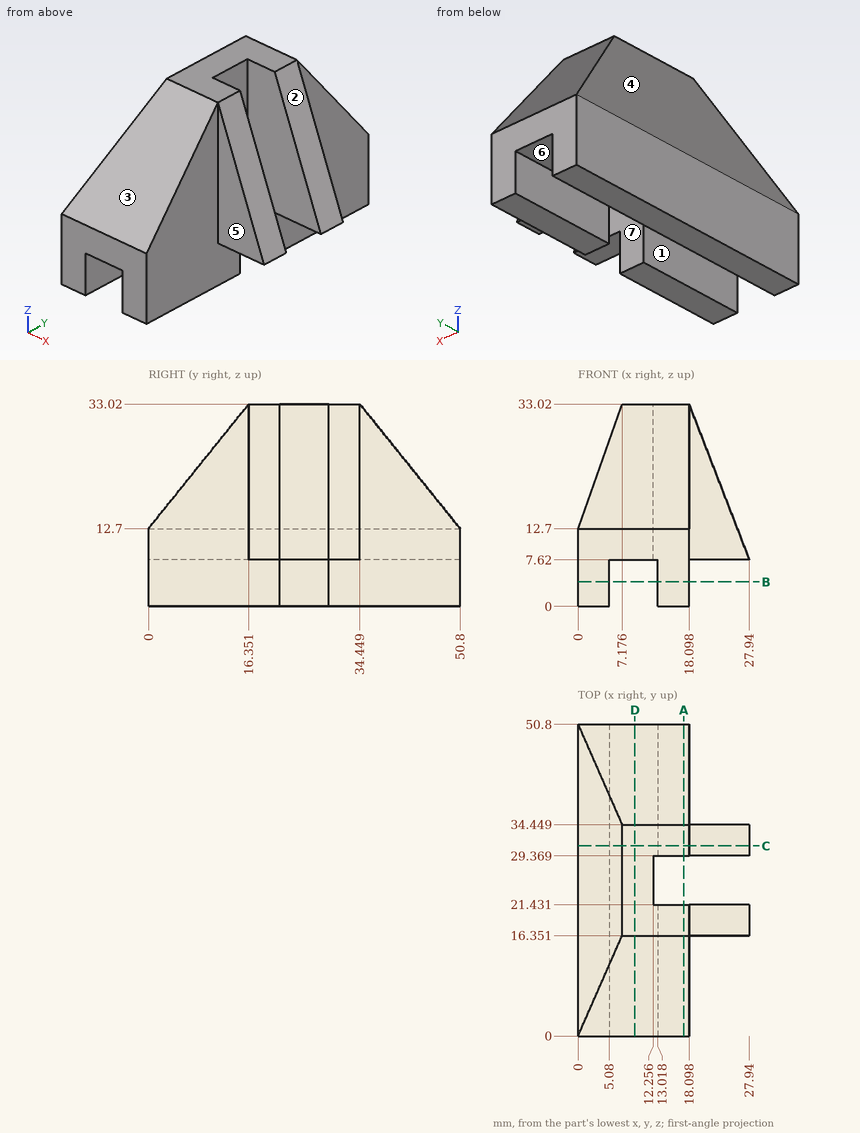
Geometry: see drawing. Coordinates: mm, zero at the bounding-box minimum. A direction names the side the tool comes from. Give positions to 0.01 mm unless a question says otherwise; leave off trailing zeros. Order: outer loops, then holes, each group sorted by start corner. A loop starts at its lowest first (then second) coordinate and runs counter-clockwise, first axis right, second up.
1. Cut plane B-B (z = 4). Return loops of the section in (x, y), and give its area (3 significant figures).
Computed:
outline: (0, 0) - (5.08, 0) - (5.08, 50.8) - (0, 50.8) - close; (13.02, 0) - (18.1, 0) - (18.1, 21.43) - (13.02, 21.43) - close; (13.02, 29.37) - (18.1, 29.37) - (18.1, 50.8) - (13.02, 50.8) - close
area: 476 mm2
2. Cut plane A-A (x = 17.25). Return loops of the section in (y, z).
Computed:
outline: (0, 0) - (21.43, 0) - (21.43, 33.02) - (16.35, 33.02) - (0, 12.7) - close; (29.37, 0) - (50.8, 0) - (50.8, 12.7) - (34.45, 33.02) - (29.37, 33.02) - close
3. Cut plane D-D (x = 9.25). Return loops of the section in (y, z).
Computed:
outline: (0, 7.62) - (50.8, 7.62) - (50.8, 12.7) - (34.45, 33.02) - (16.35, 33.02) - (0, 12.7) - close
4. Cut plane C-C (y = 31). Return loops of the section in (x, z) (1 decimal).
Computed:
outline: (0, 0) - (5.1, 0) - (5.1, 7.6) - (13, 7.6) - (13, 0) - (18.1, 0) - (18.1, 7.6) - (27.9, 7.6) - (18.1, 33) - (7.2, 33) - (0, 12.7) - close
5. Draft query along X for the marked faces 1, 2, 3 and 4. Return one class per face: released by +X, released by -X, zero draft, split by the parting line, or undercut.
Computed:
face 1: undercut
face 2: released by +X
face 3: zero draft
face 4: released by -X
6. Pin query (flat end, axial travel): pin 1 Ø5.5 at (x, y) = (24, 18) entering from -Z; pin 2 Ø10.5 at (y, z) = (42.5, 13) entering from +X; pin 3 Ø11 at (x, z) = (21.5, 22) entering from +Y (1 decimal). Return the tip coordinate at first contact, or that it passes through.
Computed:
pin 1: stops at z = 7.62
pin 2: stops at x = 18.1
pin 3: stops at y = 46.8
7. Set-up query: the marked faces 5, 6 and 7. Return all of +Z, -Z, +X, -X, +Y, -Y with unobstructed straight access to the full face (end or side cutting, diameter ignored); none if empty.
Computed:
face 5: +Z, -Z, +X, -Y
face 6: -Z, +Y, -Y
face 7: +Z, -Z, +X
8. Line query: probe 1 along Y at (x, z) = (19, 20); probe 2 along X at (y, z) = (26.5, 6); probe 3 along Z at (x, y) = (7.25, 34). Output: solid intervals per line, ascending.
Computed:
probe 1: y = 16.35 to 21.43, 29.37 to 34.45
probe 2: x = 0 to 5.08
probe 3: z = 7.62 to 33.02
